For this review, take the finished solid that the model builds, in its own axes (mm). A direction names the side the tool comes from. Give positions to 0.01 mm unless a question says otherwise; leave off trailing zeros. Write each loop counter-clockwise with the first axis right and the second up, starting at its lowest first coordinate (ties: lowest second). Pieces come first, ordered by that corner, then holes. Notation, with made-up numbers: (54, -22.75) -> (93, -22.75) arc R23 cw to (93, 6.25) -> close; hole circle Ø5 at (-38.75, 72). An arc over 180 degrees is marked (long way). Answer as CSV lines item,"result".
Autodesk Inventor part; units mm, degrees
ref_plane "Start plane" through (0, 0, 0) normal (0, 0, 1) x (1, 0, 0)
ref_plane "End plane" through (0, 0, 1219.2) normal (0, 0, 1) x (1, 0, 0)
ref_plane "Work Plane4" through (0, 0, 1219.2) normal (0.7071, 0, 0.7071) x (0.7071, 0, -0.7071)
ref_plane "Start plane" through (0, 0, 0) normal (0, 0, 1) x (1, 0, 0)
ref_plane "End plane" through (0, 0, 1219.2) normal (0, 0, 1) x (1, 0, 0)
sketch "Sketch" plane through (0, 0, 0) normal (0, 0, 1) x (1, 0, 0)
  line L0 (0, 0) -> (0, 50.8)
  line L1 (0, 50.8) -> (40.2336, 50.8)
  line L2 (40.2336, 50.8) -> (40.2336, 46.3293)
  line L3 (38.1154, 44.0972) -> (11.035, 42.6782)
  line L4 (4.6736, 35.9747) -> (4.6736, 0)
  line L5 (4.6736, 0) -> (0, 0) construction
  line L6 (22.5508, 50.8) -> (22.5508, 43.2816) construction
  line L7 (40.2336, 44.2082) -> (40.2336, 43.2816) construction
  line L8 (40.2336, 43.2816) -> (22.5508, 43.2816) construction
  line L9 (0, 15) -> (0, -27) construction
  line L10 (-5.539, 0) -> (16.0067, 0) construction
  line L11 (0, 0) -> (0, -50.8)
  line L12 (0, -50.8) -> (40.2336, -50.8)
  line L13 (40.2336, -50.8) -> (40.2336, -46.3293)
  line L14 (38.1154, -44.0972) -> (11.035, -42.6782)
  line L15 (4.6736, -35.9747) -> (4.6736, 0)
  arc A0 (11.035, 42.6782) -> (4.6736, 35.9747) centre (11.3862, 35.9747) ccw
  arc A1 (4.6736, -35.9747) -> (11.035, -42.6782) centre (11.3862, -35.9747) ccw
  arc A2 (38.1154, 44.0972) -> (40.2336, 46.3293) centre (37.9984, 46.3293) ccw
  arc A3 (40.2336, -46.3293) -> (38.1154, -44.0972) centre (37.9984, -46.3293) ccw
  line L16 (0, 71.12) -> (0, -71.12) construction
  line L17 (-14.7825, 0) -> (49.9224, 0) construction
  point P0 (4.6736, 42.3448)
  point P1 (40.2336, -44.2082)
  point P2 (4.6736, -42.3448)
  point P3 (22.5508, -50.8)
  point P4 (22.5508, -43.2816)
  dimension "d0" = 4.6736
  dimension "d1" = 50.8
  dimension "d2" = 40.2336
  dimension "d3" = 7.5184
  dimension "d4" = 17.6828
  dimension "d5" = 0.9266
  dimension "d25" = 0
  dimension "d28" = 6.7127
  dimension "d29" = 2.2352
extrude "Body" add sketch "Sketch" along normal up to surface (1219.2 mm away) from surface at 0
sketch "Sketch3" plane through (0, 0, 0) normal (0, 0, 1) x (1, 0, 0)
  line L0 (0, 0) -> (10, 0)
ref_plane "Work Plane3" through (0, 0, 0) normal (0, -1, 0) x (1, 0, 0)
sketch "Sketch4" plane through (0, 0, 0) normal (0, -1, 0) x (1, 0, 0)
  line L0 (-2, 0) -> (12, 0)
  line L1 (-2, 1219.2) -> (12, 1219.2)
  dimension "d31" = 1219.2
ref_plane "Work Plane4" through (0, 0, 1219.2) normal (0.7071, 0, 0.7071) x (0.7071, 0, -0.7071)
split "Split1" plane through (0, 0, 1219.2) removes the side toward (0.7071, 0, 0.7071)
ref_plane "Work Plane5" through (0, 0, 0) normal (0.7071, 0, -0.7071) x (-0.7071, 0, -0.7071)
split "Split2" plane through (0, 0, 0) removes the side toward (0.7071, 0, -0.7071)
equation "\"d0\" = G_T"
equation "\"d1\" = 0.5 * G_H"
equation "\"d2\" = G_W"
equation "\"d3\" = G_T1"
equation "\"d4\" = G_C"
equation "\"d28\" = G_IR"
equation "\"d29\" = G_ER"
equation "\"d6\" = G_L"
equation "\"G_W\" = 40.2336"
equation "\"G_H\" = 101.6"
equation "\"G_T\" = 4.6736"
equation "\"G_T1\" = 7.5184"
equation "\"G_NG\" = 0.0524"
equation "\"G_ER\" = 2.2352"
equation "\"G_IR\" = 6.71265"
equation "\"G_C\" = 17.68285"
equation "\"G_L\" = d31"
equation "\"ex\" = 0"
equation "\"G_OFFSET_START\" = 0"
equation "\"G_OFFSET_END\" = 0"
equation "\"d27\" = G_OFFSET_END + B_L"
equation "\"B_L\" = 1219.2"
properties part number "AISC - C 4 x 5.4 - 48" material "Steel, Mild"
Q1. Draft analysis for pull direction Y (two halves, no side actions). For faces 1 (the flat face through (4, 4, 4)), 2 (the flat face through (4.674, 1, 601)), 3 (the flat face through (20, -50.8, 601)), 4 (the flat face through (24.8, 43.4, 601.2)), state which applies: released by +Y, released by -Y, zero draft, split by the parting line, or undercut.
Answer block:
face 1,"zero draft"
face 2,"undercut"
face 3,"released by -Y"
face 4,"undercut"
Q2. To check wall thickness, follow probe 1 along Y at (x, z) = (13, 137); probe 2 along Y at (x, z) = (36.5, 1113.5); probe 3 along X at (y, z) = (37, 622). State the ranges of each line that lie inside material, in increasing order. Write a range as [from, to].
Answer block:
probe 1,"y = [-50.8, -42.78], [42.78, 50.8]"
probe 2,"y = [-50.8, -44.01], [44.01, 50.8]"
probe 3,"x = [0, 4.75]"
Q3. For faces 5 (the flat face through (24.8, -43.4, 601.2)), 6 (the flat face through (3.6, -4, 1215.6)), list the 3-axis set-ups (+Z, -Z, +X, -X, +Y, -Y) from which the entire face can be reached by the end or side of a thin tool; tool diameter is ignored.
Answer block:
face 5,"+Z, -Z, +X"
face 6,"+Z, +X, +Y, -Y"
Q4. Add section C-C (y = 9). Write out the cut boundary in (x, z).
Answer block:
outline,"(0, 0) -> (4.67, 4.67) -> (4.67, 1214.53) -> (0, 1219.2) -> close"
Q5. Clearance check with a flat-ended pin moving along its axis: pin 1 (8 mm diameter, centred on y = -29, z = 359, fed in from +X). State where the tip first meets the part, or that it passes through.
Answer block:
pin 1,"stops at x = 4.67"
Q6. Add section B-B (x = 25.5). Write out the cut boundary in (y, z).
Answer block:
outline,"(-50.8, 25.5) -> (-43.44, 25.5) -> (-43.44, 1193.7) -> (-50.8, 1193.7) -> close; (43.44, 25.5) -> (50.8, 25.5) -> (50.8, 1193.7) -> (43.44, 1193.7) -> close"
Q7. Add section A-A (z = 1111). Write out the cut boundary in (x, y) (3 decimals), plus the area to 3 significant figures.
Answer block:
outline,"(0, -50.8) -> (40.234, -50.8) -> (40.234, -46.329) arc R2.235 ccw to (38.115, -44.097) -> (11.035, -42.678) arc R6.713 cw to (4.674, -35.975) -> (4.674, 35.975) arc R6.713 cw to (11.035, 42.678) -> (38.115, 44.097) arc R2.235 ccw to (40.234, 46.329) -> (40.234, 50.8) -> (0, 50.8) -> close"
area,"1,030 mm2"
